Source: three-view drawing plus pictorial views. Frame: mm from the lowest corner of the part. A direction names the side the tool comes from. Coordinates: 2 decimals unless noted, no trailing zeros. Write each loop counter-clockwise with the first axis right and the second up, starting at its lowest first coordinate (ties: lowest second). Pieces come first, ordered by that corner, then holes. Notation, with made-up numbers: (-10.5, -2.75) - (9.5, -2.75) arc R18 cw to (9.5, 9.25) - close; hole circle Ø10 at (84.5, 52.5). An arc over 180 degrees is marked (long way). Answer as a JSON object with one key per item and string values. Group by question number.
Item 1: Section B-B on z = 22.5. Return loops of the section in (x, y) (1 decimal), and give its area (3 significant figures).
Item 2: Section A-A on y = 41.5. Return loops of the section in (x, z) (1 decimal).
Item 3: Set-up query: the marked faces 1, 2 and 3. Return all of +Z, -Z, +X, -X, +Y, -Y with unobstructed straight access to the full face (end or side cutting, diameter ignored); none if empty.
Item 4: Mould query, pull axis Y, two halves, no side actions, for the marked faces 4, 5 and 6. Classes: pulls with the +Y half, pulls with the -Y half, needs draft (parallel to the pull), parting line crosses it, or undercut.
Item 5: Section C-C on y = 27. Return loops of the section in (x, z) (1 decimal).
Item 6: Line query: line 1 along X through (y, z) = (89, 8.5); line 2 along Z through (x, y) = (95, 29) (1 decimal); line 3 along X through (y, z) = (55.5, 16). Output: solid intervals per line, ascending. Write a range as from..to.
Item 7: First-contact query: pin 1 Ø6 at (x, y) = (112, 17.5) entering from +Z (1 decimal); pin 2 Ø12 at (x, y) = (37, 94.5) entering from +Z; pin 3 Ø5 at (x, z) = (74, 34) entering from +Y (1 decimal). Flat tips, straight axial feed; report the tip coordinate or a pass-through.
Item 8: Section D-D on z = 48.5. Return loops of the section in (x, y) (1 decimal), and give its area (3 significant figures).
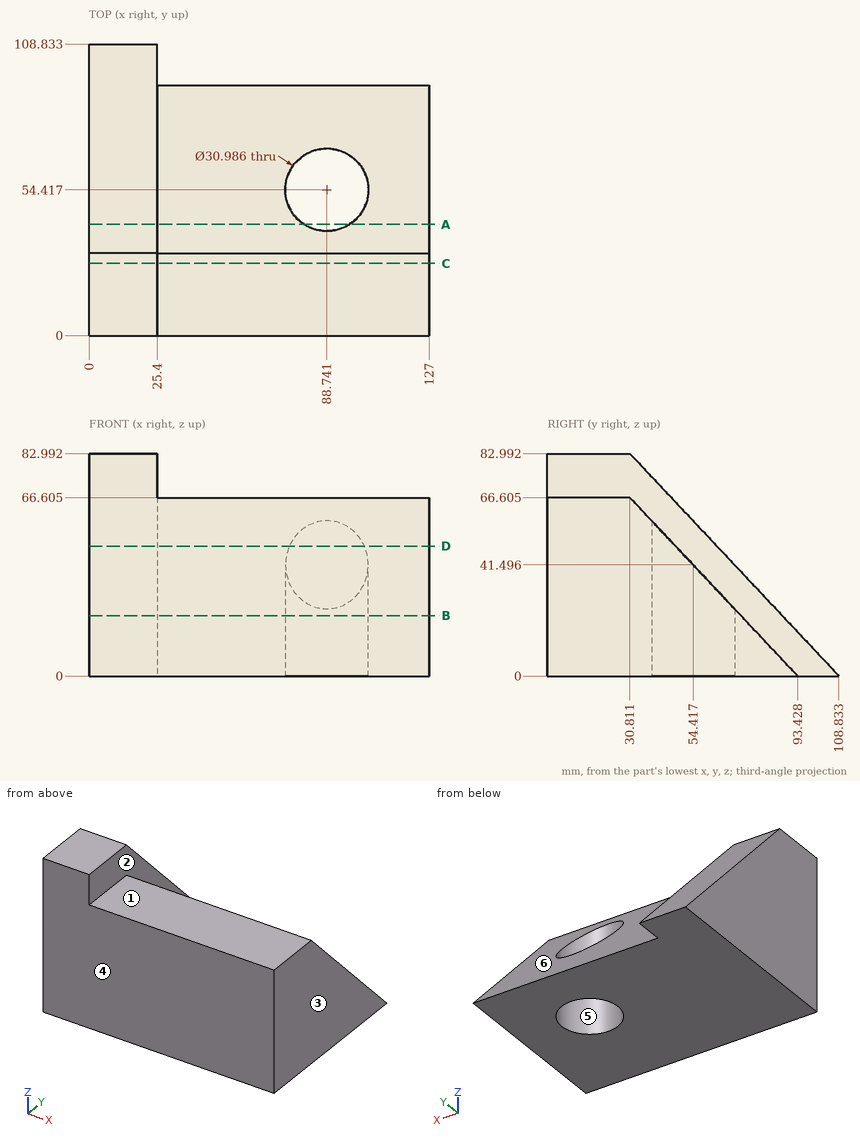
Checks:
{
 "1": {"outline": "(0, 0) - (127, 0) - (127, 72.3) - (25.4, 72.3) - (25.4, 87.7) - (0, 87.7) - close; hole circle Ø31 at (88.7, 54.4)", "area": "8,820 mm^2"},
 "2": {"outline": "(0, 0) - (80.2, 0) - (80.2, 55.2) - (25.4, 55.2) - (25.4, 71.6) - (0, 71.6) - close; (97.3, 0) - (127, 0) - (127, 55.2) - (97.3, 55.2) - close"},
 "3": {"face 1": "+Z, +X, +Y, -Y", "face 2": "+Z, +X, +Y", "face 3": "+Z, -Z, +X, +Y, -Y"},
 "4": {"face 4": "pulls with the -Y half", "face 5": "undercut", "face 6": "pulls with the +Y half"},
 "5": {"outline": "(0, 0) - (127, 0) - (127, 66.6) - (25.4, 66.6) - (25.4, 83) - (0, 83) - close"},
 "6": {"line 1": "0..25.4", "line 2": "0..66.6", "line 3": "0..73.29, 104.2..127"},
 "7": {"pin 1": "z = 66.6", "pin 2": "z = 5.24", "pin 3": "y = 63.8"},
 "8": {"outline": "(0, 0) - (127, 0) - (127, 47.8) - (102.8, 47.8) arc R15.5 cw to (74.7, 47.8) - (25.4, 47.8) - (25.4, 63.2) - (0, 63.2) - close", "area": "6,290 mm^2"}
}
